Model file for the job. Use its own axes, mm. Face numbers are marked on the shaded views. Give positions to 0.01 mm unless a question says otherwise; leave off trailing zeros. Write each loop counter-clockwise with the first axis right and the second up, starting at its lowest first coordinate (ties: lowest second). Pieces come first, ordered by that corner, then holes.
```python
from build123d import *

# Parameters (mm, degrees)
F0_W     = 107.95
F0_H     = 107.95
F1_DEPTH = 9.525
F2_W     = 104.15524
F2_H     = 104.15524
F3_DEPTH = 7.62762
F4_R     = 3.175
F6_D     = 4.0386
F6_DEPTH = 8.89
F6_TIP   = 1.213317848


with BuildPart() as f1:
    # F0 (on Top) → F1 (new body)
    with BuildSketch(Plane.XY):
        Rectangle(F0_W, F0_H)
    extrude(amount=F1_DEPTH)

    # F2 (on face) → F3 (cut)
    with BuildSketch(Plane(origin=(0, 0, 0), x_dir=(1, 0, 0), z_dir=(0, 0, -1))):
        Rectangle(F2_W, F2_H)
    extrude(amount=-F3_DEPTH, mode=Mode.SUBTRACT)

    # F4
    f4_edges = [f1.edges().sort_by_distance(p)[0] for p in [
        (0, -52.07762, 7.62762),
        (-52.07762, 0, 7.62762),
        (0, 52.07762, 7.62762),
        (52.07762, 0, 7.62762),
        (0, 53.975, 9.525),
        (-53.975, 0, 9.525),
        (0, -53.975, 9.525),
        (53.975, 0, 9.525),
    ]]
    fillet(f4_edges, radius=F4_R)

    # F6
    with Locations(Plane.XY.offset(9.525)):
        with Locations((-48.5775, 0), (48.5775, 0)):
            Hole(F6_D / 2, depth=F6_DEPTH)
            with Locations((0, 0, -(F6_DEPTH + F6_TIP / 2))):  # 118° drill point
                Cone(0, F6_D / 2, F6_TIP, mode=Mode.SUBTRACT)


solid = f1.part
```
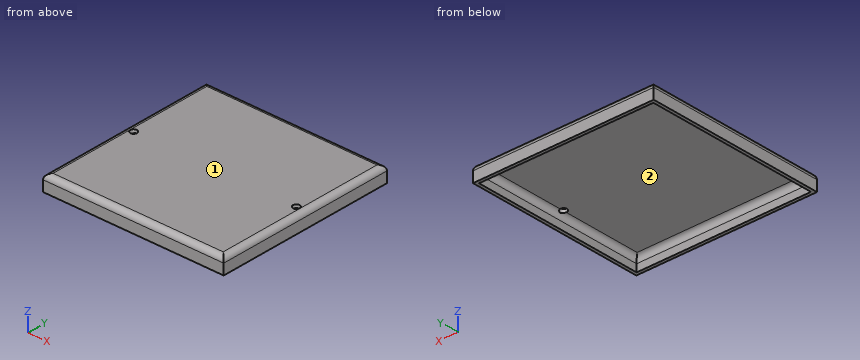
1. Probe probe 1 along X at (y, z) = (-9, 2.75) (3 decimals); probe 2 along X at (y, z) = (0, 8.4). List the from-to ranges inside material, lowest first.
Calculated:
probe 1: x = -53.975 to -52.078, 52.078 to 53.975
probe 2: x = -53.22 to -50.6, -46.56 to 46.56, 50.6 to 53.22
2. Slice it at A-A, the plane y = 0. Write the cut outline in (x, z) (3 decimals).
Calculated:
outline: (-53.975, 0) - (-52.078, 0) - (-52.078, 4.453) arc R3.175 cw to (-50.597, 7.138) - (-50.597, 9.525) - (-50.8, 9.525) arc R3.175 ccw to (-53.975, 6.35) - close; (-46.558, 7.628) - (46.558, 7.628) - (46.558, 9.525) - (-46.558, 9.525) - close; (50.597, 7.138) arc R3.175 cw to (52.078, 4.453) - (52.078, 0) - (53.975, 0) - (53.975, 6.35) arc R3.175 ccw to (50.8, 9.525) - (50.597, 9.525) - close
3. Pin check, flat tip, straight feed: P1, Ø8, axis at x = -5, y = 42, coming from the -Z side. Stop position of the tip, or through.
Calculated:
P1: stops at z = 7.63
4. Slice it at B-B, the plane y = 15. Write the cut outline in (x, z) (3 decimals), and give its area (3 significant figures).
Calculated:
outline: (-53.975, 0) - (-52.078, 0) - (-52.078, 4.453) arc R3.175 cw to (-48.903, 7.628) - (48.903, 7.628) arc R3.175 cw to (52.078, 4.453) - (52.078, 0) - (53.975, 0) - (53.975, 6.35) arc R3.175 ccw to (50.8, 9.525) - (-50.8, 9.525) arc R3.175 ccw to (-53.975, 6.35) - close
area: 234 mm2
5. Pull direction Y, two halves, no side cores. Call the marked faces 1 and 2: +Y half, -Y half, draft (parallel to the pull), parting line (faces both ways), or undercut.
Calculated:
face 1: draft
face 2: undercut
